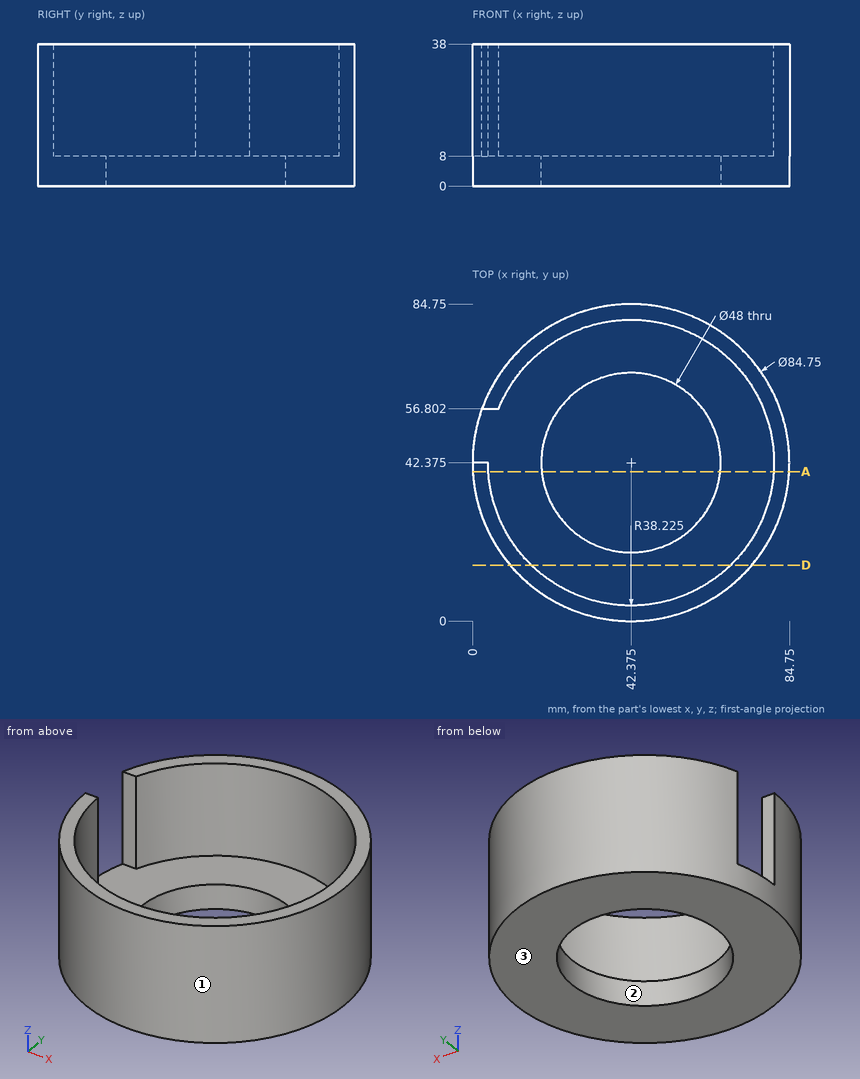
Design review of the part shown in the three views and the two pictorial views. Dimensions are in mm from the part's minimum x, y and z. Round coordinates to 2 decimals unless told otherwise and drop trailing zeros. Write each loop counter-clockwise with the first axis right and the second up, starting at its lowest first coordinate (ties: lowest second). Pieces come first, ordered by that corner, then holes. Notation, with made-up numbers: (11, 14) -> (40, 14) arc R28 ccw to (40, 38) -> close; hole circle Ø4 at (-37.75, -21.5). An arc over 180 degrees is marked (long way). One line per question, with ' | ' between items. Start each with the question number.
1) Mouldability with a two-part tool opening along Y and no side actions: class the marked faces 1, 2 and 3 as +Y half, -Y half, draft (parallel to the pull), parting line (faces both ways), or undercut.
2) Add section A-A (y = 40). Write out the cut boundary in (x, z).
3) For pin 1 Ø10 at (x, z) = (31.5, 23.5) entering from -Y; pin 2 Ø8 at (x, z) = (73.5, 16.5) entering from +Y; pin 3 Ø1 at (x, z) = (37.5, 32) entering from +Y, all flat-tipped, find the tip position at first contact; note any pin that passes through.
4) Wall thickness on line 1 along X through (y, z) = (58, 35) (1 decimal); line 2 along Y through (x, z) = (30.5, 2.5); line 3 along X through (y, z) = (8, 18) (1 decimal): over which ranges is each line inside the solid? List them lowest first.
5) Add section D-D (y = 15). Write out the cut boundary in (x, z).
Reported:
1) face 1: parting line | face 2: undercut | face 3: draft
2) outline: (0.07, 0) -> (18.49, 0) -> (18.49, 8) -> (4.22, 8) -> (4.22, 38) -> (0.07, 38) -> close; (66.26, 0) -> (84.68, 0) -> (84.68, 38) -> (80.53, 38) -> (80.53, 8) -> (66.26, 8) -> close
3) pin 1: stops at y = 0.41 | pin 2: stops at y = 74.93 | pin 3: stops at y = 84.52
4) line 1: x = 3 to 7.5, 77.3 to 81.8 | line 2: y = 1.7 to 21.52, 63.23 to 83.05 | line 3: x = 17.6 to 25.7, 59.1 to 67.2
5) outline: (10.03, 0) -> (74.72, 0) -> (74.72, 38) -> (69.05, 38) -> (69.05, 8) -> (15.7, 8) -> (15.7, 38) -> (10.03, 38) -> close
